```python
from build123d import *

# Parameters (mm, degrees)
SKETCH6_R               = 2.1
BOSS_EXTRUDE1_DEPTH     = 310
SKETCH7_R               = 4.5
CUT_EXTRUDE1_DEPTH      = 11
CUT_EXTRUDE1_DEPTH_BACK = 11


with BuildPart() as part:
    # Sketch6 → Boss-Extrude1 (new body)
    with BuildSketch(Plane.XY):
        with BuildLine():
            Line((-3.4, -2.339339828), (-3.4, 2.339339828))
            Line((-3.4, 2.339339828), (-6.560660172, 5.5))
            Line((-6.560660172, 5.5), (-8.2, 5.5))
            Line((-8.2, 5.5), (-8.2, 2.89))
            Line((-8.2, 2.89), (-8.31, 2.89))
            Line((-8.31, 2.89), (-9.768614357, 4.348614357))
            ThreePointArc((-9.768614357, 4.348614357), (-9.939864831, 4.604908803), (-10, 4.907228714))
            Line((-10, 4.907228714), (-10, 8.5))
            ThreePointArc((-10, 8.5), (-9.560660172, 9.560660172), (-8.5, 10))
            Line((-8.5, 10), (-4.907228714, 10))
            ThreePointArc((-4.907228714, 10), (-4.604908803, 9.939864831), (-4.348614357, 9.768614357))
            Line((-4.348614357, 9.768614357), (-2.89, 8.31))
            Line((-2.89, 8.31), (-2.89, 8.2))
            Line((-2.89, 8.2), (-5.5, 8.2))
            Line((-5.5, 8.2), (-5.5, 6.560660172))
            Line((-5.5, 6.560660172), (-2.339339828, 3.4))
            Line((-2.339339828, 3.4), (2.339339828, 3.4))
            Line((2.339339828, 3.4), (5.5, 6.560660172))
            Line((5.5, 6.560660172), (5.5, 8.2))
            Line((5.5, 8.2), (2.89, 8.2))
            Line((2.89, 8.2), (2.89, 8.31))
            Line((2.89, 8.31), (4.348614357, 9.768614357))
            ThreePointArc((4.348614357, 9.768614357), (4.604908803, 9.939864831), (4.907228714, 10))
            Line((4.907228714, 10), (8.5, 10))
            ThreePointArc((8.5, 10), (9.560660172, 9.560660172), (10, 8.5))
            Line((10, 8.5), (10, 4.907228714))
            ThreePointArc((10, 4.907228714), (9.939864831, 4.604908803), (9.768614357, 4.348614357))
            Line((9.768614357, 4.348614357), (8.31, 2.89))
            Line((8.31, 2.89), (8.2, 2.89))
            Line((8.2, 2.89), (8.2, 5.5))
            Line((8.2, 5.5), (6.560660172, 5.5))
            Line((6.560660172, 5.5), (3.4, 2.339339828))
            Line((3.4, 2.339339828), (3.4, -2.339339828))
            Line((3.4, -2.339339828), (6.560660172, -5.5))
            Line((6.560660172, -5.5), (8.2, -5.5))
            Line((8.2, -5.5), (8.2, -2.89))
            Line((8.2, -2.89), (8.31, -2.89))
            Line((8.31, -2.89), (9.768614357, -4.348614357))
            ThreePointArc((9.768614357, -4.348614357), (9.939864831, -4.604908803), (10, -4.907228714))
            Line((10, -4.907228714), (10, -8.5))
            ThreePointArc((10, -8.5), (9.560660172, -9.560660172), (8.5, -10))
            Line((8.5, -10), (4.907228714, -10))
            ThreePointArc((4.907228714, -10), (4.604908803, -9.939864831), (4.348614357, -9.768614357))
            Line((4.348614357, -9.768614357), (2.89, -8.31))
            Line((2.89, -8.31), (2.89, -8.2))
            Line((2.89, -8.2), (5.5, -8.2))
            Line((5.5, -8.2), (5.5, -6.560660172))
            Line((5.5, -6.560660172), (2.339339828, -3.4))
            Line((2.339339828, -3.4), (-2.339339828, -3.4))
            Line((-2.339339828, -3.4), (-5.5, -6.560660172))
            Line((-5.5, -6.560660172), (-5.5, -8.2))
            Line((-5.5, -8.2), (-2.89, -8.2))
            Line((-2.89, -8.2), (-2.89, -8.31))
            Line((-2.89, -8.31), (-4.348614357, -9.768614357))
            ThreePointArc((-4.348614357, -9.768614357), (-4.604908803, -9.939864831), (-4.907228714, -10))
            Line((-4.907228714, -10), (-8.5, -10))
            ThreePointArc((-8.5, -10), (-9.560660172, -9.560660172), (-10, -8.5))
            Line((-10, -8.5), (-10, -4.907228714))
            ThreePointArc((-10, -4.907228714), (-9.939864831, -4.604908803), (-9.768614357, -4.348614357))
            Line((-9.768614357, -4.348614357), (-8.31, -2.89))
            Line((-8.31, -2.89), (-8.2, -2.89))
            Line((-8.2, -2.89), (-8.2, -5.5))
            Line((-8.2, -5.5), (-6.560660172, -5.5))
            Line((-6.560660172, -5.5), (-3.4, -2.339339828))
        make_face()
        Circle(SKETCH6_R, mode=Mode.SUBTRACT)
        Polygon((-7.66, 6.57), (-6.57, 7.66), (-6.57, 8.2), (-8.2, 8.2), (-8.2, 6.57), align=None, mode=Mode.SUBTRACT)
        Polygon((8.2, 6.57), (7.66, 6.57), (6.57, 7.66), (6.57, 8.2), (8.2, 8.2), align=None, mode=Mode.SUBTRACT)
        Polygon((7.66, -6.57), (6.57, -7.66), (6.57, -8.2), (8.2, -8.2), (8.2, -6.57), align=None, mode=Mode.SUBTRACT)
        Polygon((-8.2, -6.57), (-7.66, -6.57), (-6.57, -7.66), (-6.57, -8.2), (-8.2, -8.2), align=None, mode=Mode.SUBTRACT)
    extrude(amount=-BOSS_EXTRUDE1_DEPTH)

    # Sketch7 → Cut-Extrude1 (cut, two sides)
    with BuildSketch(Plane(origin=(0, 0, 0), x_dir=(1, 0, 0), z_dir=(0, 1, 0))) as cut_extrude1_sk:
        with Locations((0, 52.93)):
            Circle(SKETCH7_R)
    extrude(amount=CUT_EXTRUDE1_DEPTH, mode=Mode.SUBTRACT)
    extrude(cut_extrude1_sk.sketch, amount=-CUT_EXTRUDE1_DEPTH_BACK, mode=Mode.SUBTRACT)


solid = part.part
```
Source: CAD feature listing. Evaluate the final solid. Frame: model axes, mm. A direction names the side the tool comes from. Give positions to 0.01 mm unless a question says otherwise; leave off trailing zeros.
1. Section query A-A (z = -187). Count the separate pieces of the cut face and the enclosed holes in it, then the cut area to 3 significant figures.
2. Access query for faces 1 (the face through (0, -3.4, -182)), 2 (the face through (0, 3.4, -24)), 3 (the face through (3.4, 0, -181)). Directions: +Z, -Z, +X, -X, +Y, -Y. A direction counts if a zero-diameter tool reaches every point of the face in a straight line with its end or side. Return the directions, or none.
3. Pull-direction query (X, two-part tool) for faces 4 (the face through (0.1, 2.4, 0)), 5 (the face through (0, 3.4, -182)), 6 (the face through (-3.4, 0, -181)), 7 (the face through (0, -3.4, -24)); classes: +X half, -X half, draft (parallel to the pull), parting line (faces both ways), or undercut.
4. First-contact query: pin 1 (0.8 mm diameter, centred on x = -4, z = -143.5, fed in from -Y). Flat tip, straight axial feed; report the tip coordinate or a pass-through.
5. Material intervals for line 1 along X through (y, z) = (-8, -35.5); line 2 along X through (y, z) = (4.5, -35), sorted ascending.
Output values:
1. separate pieces: 1
1. enclosed holes: 5
1. area: 152 mm2
2. face 1: +Z, -Z, -Y
2. face 2: +Z, -Z, +Y
2. face 3: +Z, -Z, +X
3. face 4: draft
3. face 5: undercut
3. face 6: -X half
3. face 7: undercut
4. pin 1: stops at y = -9.82
5. line 1: x = -10 to -8.2, -6.57 to -5.5, 5.5 to 6.57, 8.2 to 10
5. line 2: x = -9.89 to -8.2, -5.56 to -3.44, 3.44 to 5.56, 8.2 to 9.89
